Can you work these out from the drawing? Everything is in mm from the part's minimum corner. Round coordinates to 2 decimals unless told otherwise and drop trailing zeros. Write each loop counter-clockwise with the first axis right and the second up, starting at its lowest first coordinate (ties: lowest second). Pieces come first, ordered by that corner, then holes. Notation, with made-up numbers: (75.5, 44) - (134.5, 44) arc R20 ccw to (134.5, 58) - close; hole circle Ø8 at (-39, 31.25). An arc over 180 degrees is marked (long way). Write each question's results on one line, items separated by ' | '. Start each with the question number.
(1) Please list where these lines run through material, in increasing order: line 1 (Z direction, x = 2.25, y = 23); line 2 (Z direction, x = 2.1, y = 8) (1 decimal). Write a range as [from, to].
(2) Imagine slicing it at A-A on x = 2.3. Write out the boundary of the cut face in (y, z) (1 decimal), then the cut area to 3 significant figures.
(3) For P1, Ø4, axis at y = 36.5, z = 78.5, coming from the -X side, with a flat end and sliding along its axis, tell me the tip position at first contact or that it passes through.
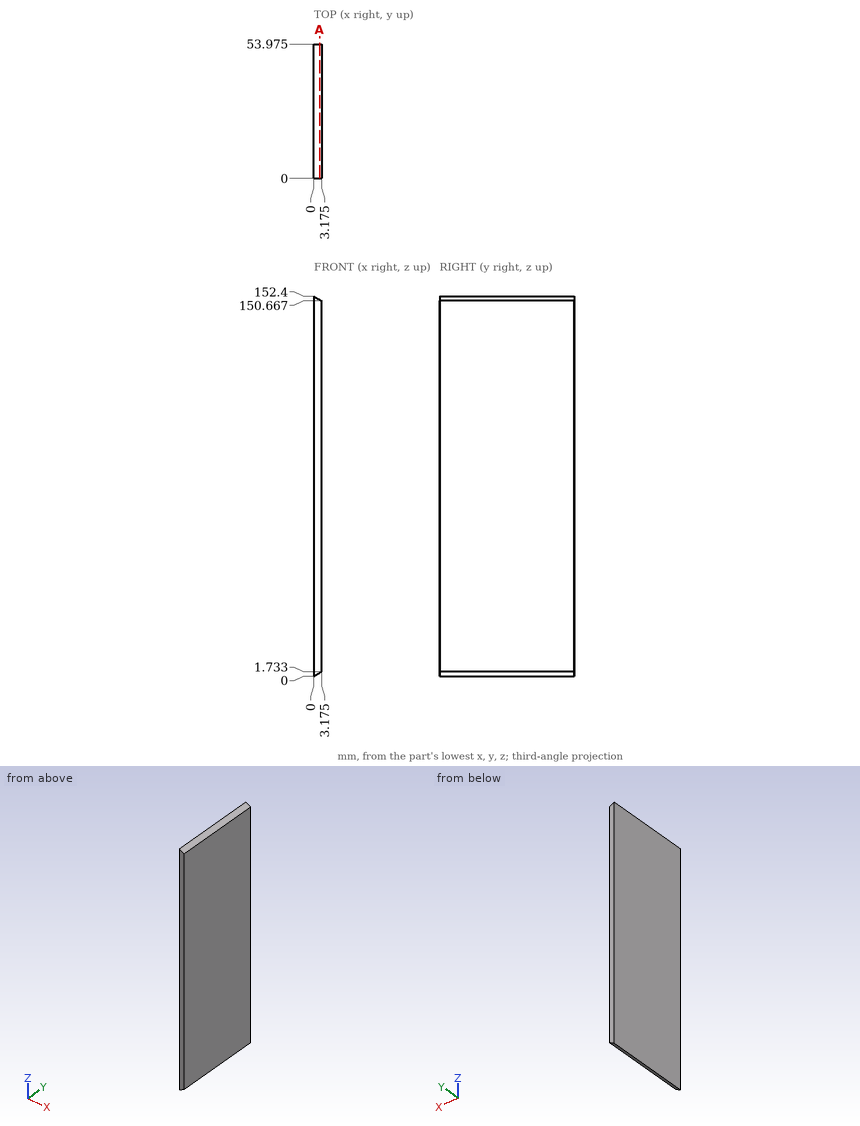
Response:
1) line 1: [1.23, 151.17] | line 2: [1.1, 151.3]
2) outline: (0, 1.3) - (54, 1.3) - (54, 151.1) - (0, 151.1) - close | area: 8,090 mm²
3) P1: x = 0
